Source: three-view drawing plus pictorial views. Frame: mm from the lowest corner of the part. Give positions to 0.01 mm unless a question says otherwise; leave off trailing zeros. Loops run counter-clockwise (first coordinate to the right, second up) from the corner with the lowest first, then second, coordinate; pieces in that order, holes last.
1. Section C-C, the plane z = 47.5. Output: boundary loops of the cut face in (x, y).
2. Material intervals for line 1 along Z through (x, y) = (58.25, 3.1); line 2 along X through (y, z) = (1.55, 47.5); line 3 along X through (y, z) = (3.8, 44), sorted ascending.
3. Section A-A, the plane z = 38.5. Output: boundary loops of the cut face in (x, y), then the cut area to 3 significant figures.
4. Section D-D, the plane x = 58.25. Output: boundary loops of the cut face in (y, z).
5. First-contact query: P1, Ø2.5, axis at x = 58.25, z = 17.5, coming from the +Y side. Flat tip, straight axial feed; report the tip coordinate or a pass-through.
6. Section B-B, the plane x = 23. Output: boundary loops of the cut face in (y, z).
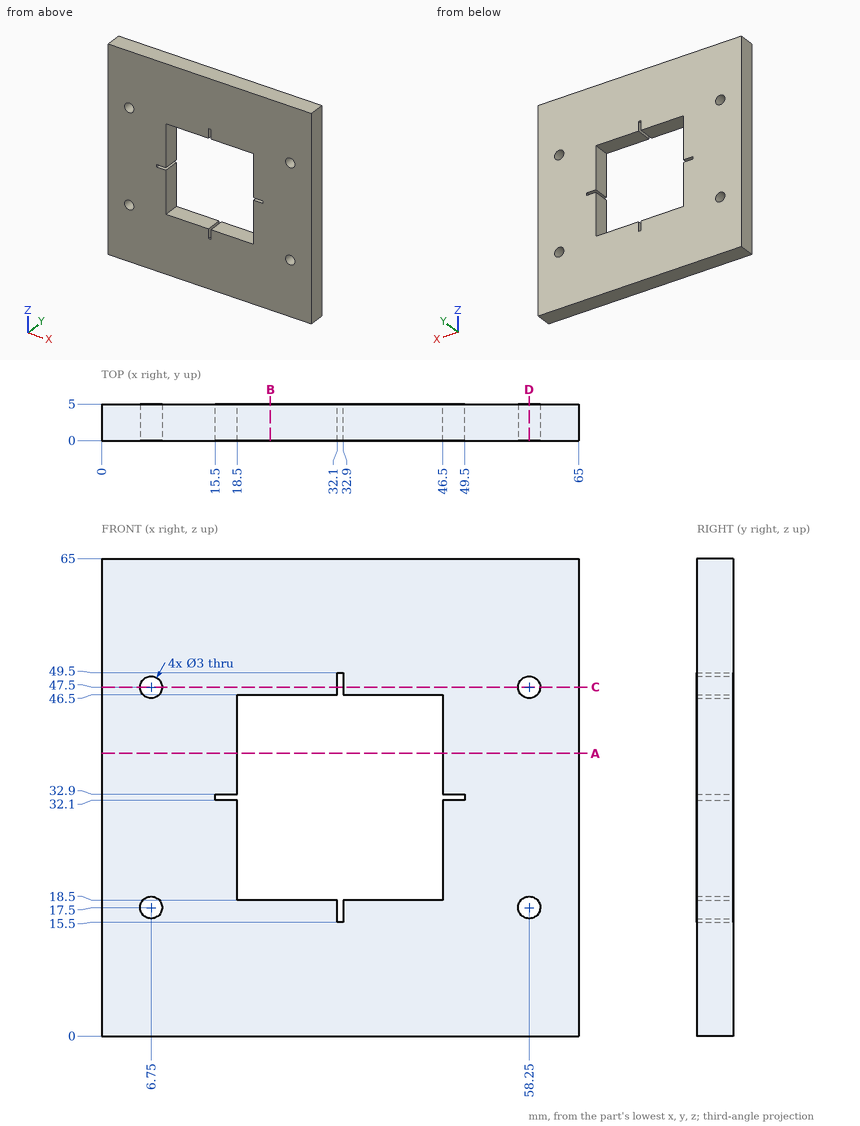
Answers below:
1. outline: (0, 0) - (5.25, 0) - (5.25, 5) - (0, 5) - close; (8.25, 0) - (32.1, 0) - (32.1, 5) - (8.25, 5) - close; (32.9, 0) - (56.75, 0) - (56.75, 5) - (32.9, 5) - close; (59.75, 0) - (65, 0) - (65, 5) - (59.75, 5) - close
2. line 1: z = 0 to 16, 19 to 46, 49 to 65
2. line 2: x = 0 to 5.25, 8.25 to 32.1, 32.9 to 56.75, 59.75 to 65
2. line 3: x = 0 to 18.5, 46.5 to 65
3. outline: (0, 0) - (18.5, 0) - (18.5, 5) - (0, 5) - close; (46.5, 0) - (65, 0) - (65, 5) - (46.5, 5) - close
3. area: 185 mm2
4. outline: (0, 0) - (5, 0) - (5, 16) - (0, 16) - close; (0, 19) - (5, 19) - (5, 46) - (0, 46) - close; (0, 49) - (5, 49) - (5, 65) - (0, 65) - close
5. P1: passes through
6. outline: (0, 0) - (5, 0) - (5, 18.5) - (0, 18.5) - close; (0, 46.5) - (5, 46.5) - (5, 65) - (0, 65) - close
